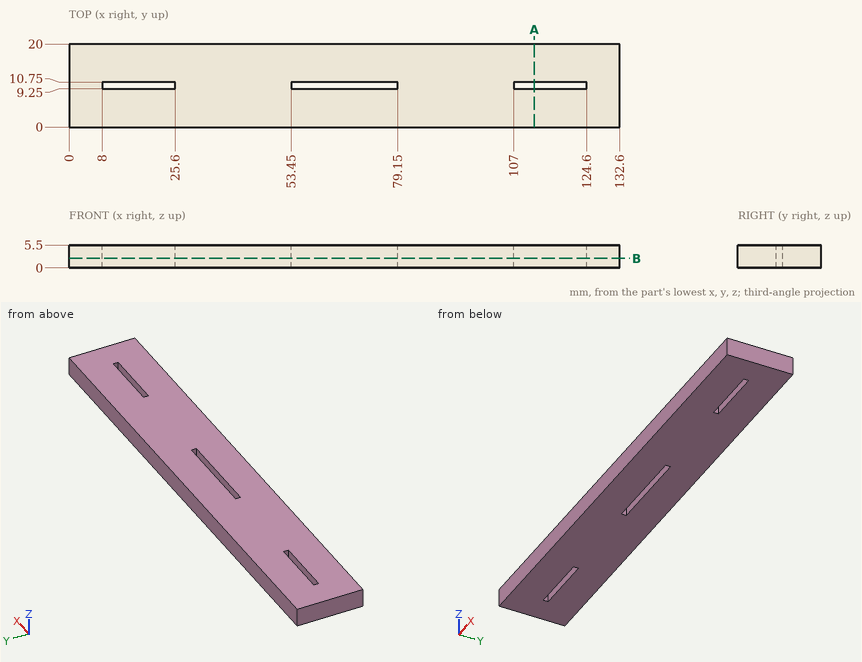
Design review of the part shown in the three views and the two pictorial views. Dimensions are in mm from the part's minimum x, y and z. Give positions to 0.01 mm unless a question says otherwise; leave off trailing zeros. Loops run counter-clockwise (first coordinate to the right, second up) from the corner with the lowest first, then second, coordinate; pieces in that order, holes last. Notation, with made-up numbers: (2, 41) -> (10, 41) arc R34 cw to (10, 76) -> close; hole circle Ø6 at (21, 85). An arc over 180 degrees is marked (long way). Put each result on its own line as item: value. Start each with the question number.
1. Wall thickness on probe 1 along X at (y, z) = (9.5, 4.35); probe 2 along Y at (x, z) = (60.5, 1.2): over which ranges is each line inside the solid? List them lowest first.
2. We need section A-A on x = 112. State the section outline as (y, z) points, then the cut area to 3 significant figures.
3. We need section B-B on z = 2.3. State the section outline as (x, y) points.
Determined:
1. probe 1: 0 to 8, 25.6 to 53.45, 79.15 to 107, 124.6 to 132.6
1. probe 2: 0 to 9.25, 10.75 to 20
2. outline: (0, 0) -> (9.25, 0) -> (9.25, 5.5) -> (0, 5.5) -> close; (10.75, 0) -> (20, 0) -> (20, 5.5) -> (10.75, 5.5) -> close
2. area: 102 mm^2
3. outline: (0, 0) -> (132.6, 0) -> (132.6, 20) -> (0, 20) -> close; hole (8, 9.25) -> (25.6, 9.25) -> (25.6, 10.75) -> (8, 10.75) -> close; hole (53.45, 9.25) -> (79.15, 9.25) -> (79.15, 10.75) -> (53.45, 10.75) -> close; hole (107, 9.25) -> (124.6, 9.25) -> (124.6, 10.75) -> (107, 10.75) -> close
